Here's how the part is built. I have some questions about the finished solid (model axes, mm). A direction names the side the tool comes from. Give positions to 0.01 mm unless a question says otherwise; leave off trailing zeros. Loops run counter-clockwise (first coordinate to the right, second up) from the corner with the lowest first, then second, coordinate; pieces in that order, holes last.
Q1. For faces 1 (the face through (-12.465, 56.133, 13.293)), 2 (the face through (26.5, -12.8, 0)), which set-ups out of +Z, -Z, +X, -X, +Y, -Y let a thin tool reach every point of the face, with its end or its side?
Q2. Suppose I cut it at D-D (y = 48.5). List the corners of the cut face in (x, z) for me.
Q3. Suppose I cut it at A-A (x = 0). List the corners of the cut face in (y, z) for me, and give its area (3 significant figures).
Q4. I'm going to push flat-ended pins straight in: P1, Ø8, axis at x = -49, z = 13.5, coming from the -Y side; P2, Ø3, axis at y = 7.5, z = 4, coming from the -X side; P3, Ø12, axis at x = -27.5, z = 19.5, coming from the +Y side. Where does each tip first touch, or does it pass through?
Q5. Suppose I cut it at B-B (z = 10.5). List the corners of the cut face in (x, y) for me.
Q6. Thinking about a two-plate mould opening in X: for faces 3 (the face through (41, -41, 22.85)), 4 (the face through (28.38, 54.56, 11.27)), 5 (the face through (-0.2, -29.2, 13.5)), which applies, pulls with the +X half, pulls with the -X half, needs draft (parallel to the pull), parting line crosses it, or undercut?
Q7. I need wall thicknesses on probe 1 along Y at (x, z) = (0, 7.5); probe 2 along X at (y, z) = (-3.5, 10); probe 3 along X at (y, z) = (30, 10.75). Which ranges of each line are inside material? Lowest first, please.
Autodesk Inventor part; units mm, degrees
ref_plane "YZ Plane" through (0, 0, 0) normal (1, 0, 0) x (0, 1, 0)
ref_plane "XZ Plane" through (0, 0, 0) normal (0, 1, 0) x (-1, 0, 0)
ref_plane "XY Plane" through (0, 0, 0) normal (0, 0, 1) x (1, 0, 0)
sketch "Sketch1" plane through (0, 0, 0) normal (0, 0, 1) x (1, 0, 0)
  circle A0 centre (0, 0) radius 61.5
  dimension "d0" = 123
extrude "Extrusion1" add sketch "Sketch1" along normal blind 4
sketch "Sketch2" plane through (0, 0, 4) normal (0, 0, 1) x (1, 0, 0)
  circle A0 centre (0, 0) radius 61.5
  circle A1 centre (0, 0) radius 57.5
  dimension "d12" = 115
extrude "Extrusion2" add sketch "Sketch2" along normal blind 18.85
sketch "Sketch3" plane through (0, 0, 0) normal (0, 0, -1) x (-1, 0, 0)
  circle A0 centre (0, 0) radius 29
  dimension "d6" = 58
extrude "Extrusion3" cut sketch "Sketch3" against normal through all
sketch "Sketch4" plane through (0, 0, 4) normal (0, 0, 1) x (1, 0, 0)
  circle A0 centre (0, 0) radius 29
  circle A1 centre (0, 0) radius 33
  dimension "d9" = 4
extrude "Extrusion4" add sketch "Sketch4" along normal blind 9.5
properties part number "stator_housing"
Solutions:
1. face 1: +Z
1. face 2: -Z, +X, -X, +Y, -Y
2. outline: (-37.82, 0) - (37.82, 0) - (37.82, 22.85) - (30.89, 22.85) - (30.89, 4) - (-30.89, 4) - (-30.89, 22.85) - (-37.82, 22.85) - close
3. outline: (-61.5, 0) - (-29, 0) - (-29, 13.5) - (-33, 13.5) - (-33, 4) - (-57.5, 4) - (-57.5, 22.85) - (-61.5, 22.85) - close; (29, 0) - (61.5, 0) - (61.5, 22.85) - (57.5, 22.85) - (57.5, 4) - (33, 4) - (33, 13.5) - (29, 13.5) - close
3. area: 487 mm2
4. P1: stops at y = -41.92
4. P2: stops at x = -61.21
4. P3: stops at y = 57.62
5. outline: circle Ø123 at (0, 0); circle Ø66 at (0, 0); hole circle Ø115 at (0, 0); hole circle Ø58 at (0, 0)
6. face 3: needs draft
6. face 4: parting line crosses it
6. face 5: undercut
7. probe 1: y = -61.5 to -57.5, -33 to -29, 29 to 33, 57.5 to 61.5
7. probe 2: x = -61.4 to -57.39, -32.81 to -28.79, 28.79 to 32.81, 57.39 to 61.4
7. probe 3: x = -53.69 to -49.05, -13.75 to 13.75, 49.05 to 53.69
